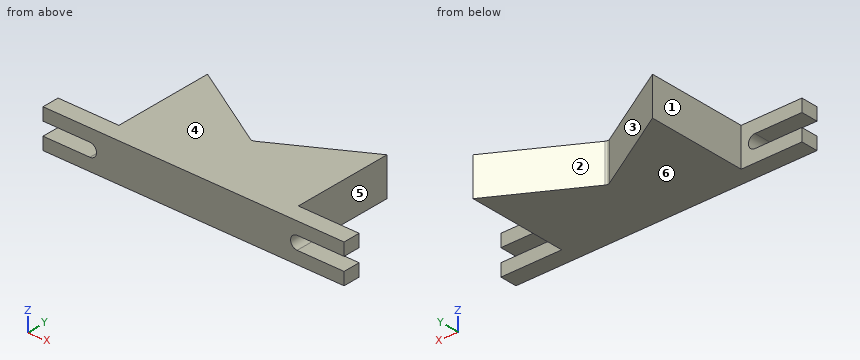
```python
from build123d import *

# Parameters (mm, degrees)
BOSS_EXTRUDE1_DEPTH = 20.7518
CUT_EXTRUDE1_DEPTH  = 10
FILLET1_R           = 2.54


with BuildPart() as part:
    # Sketch1 → Boss-Extrude1 (new body)
    with BuildSketch(Plane.XY):
        Polygon((-48.735, 28.137165369), (0, 0), (48.735, 28.137165369), (48.735, -26.443474646), (81.755, -26.443474646), (81.755, -35.714474646), (81.623037502, -35.714474646), (-81.623037502, -35.714474646), (-81.755, -35.714474646), (-81.755, -26.443474646), (-48.735, -26.443474646), align=None)
    extrude(amount=BOSS_EXTRUDE1_DEPTH)

    # Sketch2 → Cut-Extrude1 (cut)
    with BuildSketch(Plane(origin=(0, -26.443474646, 0), x_dir=(1, 0, 0), z_dir=(0, 1, 0))):
        with BuildLine():
            Line((-56.257083812, -6.8199), (-81.755, -6.8199))
            Line((-81.755, -6.8199), (-81.755, -13.9319))
            Line((-81.755, -13.9319), (-56.257083812, -13.9319))
            ThreePointArc((-56.257083812, -13.9319), (-52.701083812, -10.3759), (-56.257083812, -6.8199))
        make_face()
        with BuildLine():
            Line((81.755, -13.9319), (81.755, -6.8199))
            Line((81.755, -6.8199), (56.257083812, -6.8199))
            ThreePointArc((56.257083812, -6.8199), (52.701083812, -10.3759), (56.257083812, -13.9319))
            Line((56.257083812, -13.9319), (81.755, -13.9319))
        make_face()
    extrude(amount=-CUT_EXTRUDE1_DEPTH, mode=Mode.SUBTRACT)

    # Fillet1
    fillet1_edges = [part.edges().sort_by_distance(p)[0] for p in [
        (0, 0, 10.3759),
    ]]
    fillet(fillet1_edges, radius=FILLET1_R)


solid = part.part
```
Could you check a few things on this model? Use its own coordinates, in mm. Face numbers are marked on the shaded views. A direction names the side the tool comes from. Coordinates: 2 decimals unless noted, no trailing zeros. Write each loop counter-clockwise with the first axis right and the second up, starting at its lowest first coordinate (ties: lowest second). Pieces come first, ordered by that corner, then holes. Notation, with made-up numbers: (-6, 14) - (42, 14) arc R5 ccw to (42, 19) - close; hole circle Ø5 at (68.5, 68.5). An arc over 180 degrees is marked (long way). Use a Markdown table: item, result.
Q1. Which directions (+Z, -Z, +X, -X, +Y, -Y) give clear straight access to the entire face, cutting with the end or side of a thin tool? Please do the marked faces 5 and 6.
Geometry check:
| item | result |
|---|---|
| face 5 | +Z, -Z, +X, +Y |
| face 6 | -Z, +X, -X, +Y, -Y |
Q2. Imagine slicing it at B-B (z = 17). List the corners of the cut face in (x, y) for me (3 decimals).
Geometry check:
| item | result |
|---|---|
| outline | (-81.755, -35.714) - (81.755, -35.714) - (81.755, -26.443) - (48.735, -26.443) - (48.735, 28.137) - (1.27, 0.733) arc R2.54 cw to (-1.27, 0.733) - (-48.735, 28.137) - (-48.735, -26.443) - (-81.755, -26.443) - close |
Q3. I'm going to push flat-ended pins straight in: pin 1 Ø2 at (y, z) = (19, 8.5) entering from -X (3 decimals); pin 2 Ø2 at (y, z) = (-26, 10.5) entering from +X; pin 3 Ø4.5 at (x, y) = (75.5, -32.5) entering from -Z; pin 4 Ø1.5 at (x, z) = (-14.5, 12.5) entering from +Y. Where does each tip first touch, or does it pass through?
Geometry check:
| item | result |
|---|---|
| pin 1 | stops at x = -48.735 |
| pin 2 | stops at x = 52.85 |
| pin 3 | stops at z = 0 |
| pin 4 | stops at y = 8.8 |
Q4. Imagine slicing it at D-D (y = -12.5). List the corners of the cut face in (x, z) for me (3 decimals).
Geometry check:
| item | result |
|---|---|
| outline | (-48.735, 0) - (48.735, 0) - (48.735, 20.752) - (-48.735, 20.752) - close |
Q5. Thinking about a two-plate mould opening in X: for the marked faces 1, 2, 3 and 4, which applies, +X half, -X half, draft (parallel to the pull), parting line (faces both ways), or undercut?
Geometry check:
| item | result |
|---|---|
| face 1 | -X half |
| face 2 | undercut |
| face 3 | undercut |
| face 4 | draft |
Q6. Imagine slicing it at C-C (y = 21.5). List the corners of the cut face in (x, z) for me (3 decimals).
Geometry check:
| item | result |
|---|---|
| outline | (-48.735, 0) - (-37.239, 0) - (-37.239, 20.752) - (-48.735, 20.752) - close; (37.239, 0) - (48.735, 0) - (48.735, 20.752) - (37.239, 20.752) - close |
Q7. Imagine slicing it at A-A (x = -70.5). List the corners of the cut face in (y, z) for me, and give its area (3 significant figures).
Geometry check:
| item | result |
|---|---|
| outline | (-35.71, 0) - (-26.44, 0) - (-26.44, 6.82) - (-35.71, 6.82) - close; (-35.71, 13.93) - (-26.44, 13.93) - (-26.44, 20.75) - (-35.71, 20.75) - close |
| area | 126 mm2 |
Q8. Please list where these lines run through material, in increasing order: L1, parallel to X at y = 24.5, z = 10.5 (3 decimals); L2, parallel to X at y = 12, z = 13 (3 decimals); L3, parallel to X at y = -22, z = 16.25 (3 decimals).
Geometry check:
| item | result |
|---|---|
| L1 | x = -48.735 to -42.435, 42.435 to 48.735 |
| L2 | x = -48.735 to -20.785, 20.785 to 48.735 |
| L3 | x = -48.735 to 48.735 |
